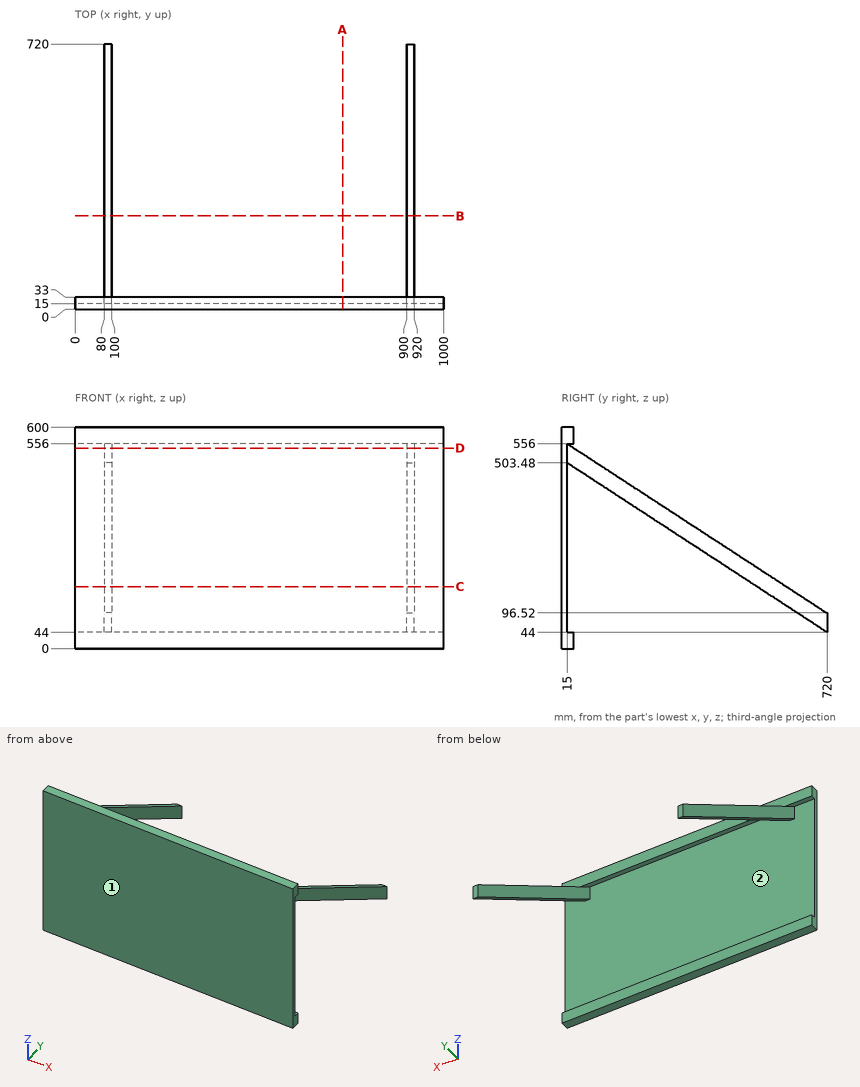
Input: dimensioned drawing with shaded views. Units: mm. Origin: part minimum x, y, z. Give positions to 0.01 mm unless a question says otherwise; leave off trailing zeros. Write each loop counter-clockwise with the first axis right and the second up, starting at its lowest first coordinate (ties: lowest second). Pieces come first, ordered by that corner, then holes. Notation, with made-up numbers: (-33.75, 83) - (3.25, 83) arc R5 cw to (3.25, 88) - close; hole circle Ø8 at (-22.5, 56.25). An arc over 180 degrees is marked (long way). Write item = value, one per line. Start each with the question number.
1) Material intervals for L1, parallel to X at y = 340, z = 308; L2, parallel to Y at x = 105, z = 197.5, sorted ascending. Write a range as [from, to].
2) Cut plane D-D (z = 543.5). Return loops of the section in (x, y).
3) Cut plane A-A (x = 726). Return loops of the section in (y, z).
4) Pin query (flat end, axial travel): pin 1 (12 mm diameter, centred on x = 323.5, z = 244, fed in from +Y). Return the tip coordinate at first contact, or that it passes through.
5) Draft query along Z for the marked faces 1 and 2. Return one class per face: pulls with the +Z half, pulls with the -Z half, needs draft (parallel to the pull), parting line crosses it, or undercut.
6) Cut plane C-C (z = 168). Return loops of the section in (x, y), and give its area (3 significant figures).
7) Cut plane B-B (y = 254). Return loops of the section in (x, z).
Answers follow:
q1.L1 = [80, 100], [900, 920]
q1.L2 = [0, 15]
q2.outline = (0, 0) - (1000, 0) - (1000, 15) - (920, 15) - (920, 34.18) - (900, 34.18) - (900, 15) - (100, 15) - (100, 34.18) - (80, 34.18) - (80, 15) - (0, 15) - close
q3.outline = (0, 0) - (33, 0) - (33, 44) - (15, 44) - (15, 556) - (33, 556) - (33, 600) - (0, 600) - close
q4.pin_1 = 15
q5.face_1 = needs draft
q5.face_2 = undercut
q6.outline = (0, 0) - (1000, 0) - (1000, 15) - (0, 15) - close; (80, 529.74) - (100, 529.74) - (100, 610.33) - (80, 610.33) - close; (900, 529.74) - (920, 529.74) - (920, 610.33) - (900, 610.33) - close
q6.area = 18,200 mm^2
q7.outline = (80, 347.71) - (100, 347.71) - (100, 400.23) - (80, 400.23) - close; (900, 347.71) - (920, 347.71) - (920, 400.23) - (900, 400.23) - close
